```python
from build123d import *

# Parameters (mm, degrees)
SKETCH1_W           = 254
SKETCH1_H           = 177.8
BOSS_EXTRUDE1_DEPTH = 127
SKETCH2_W           = 228.6
SKETCH2_H           = 152.4
CUT_EXTRUDE1_DEPTH  = 101.6


with BuildPart() as part:
    # Sketch1 → Boss-Extrude1 (new body)
    with BuildSketch(Plane(origin=(0, 0, 0), x_dir=(1, 0, 0), z_dir=(0, 1, 0))):
        Rectangle(SKETCH1_W, SKETCH1_H)
    extrude(amount=BOSS_EXTRUDE1_DEPTH)

    # Sketch2 → Cut-Extrude1 (cut)
    with BuildSketch(Plane(origin=(0, 127, 0), x_dir=(1, 0, 0), z_dir=(0, 1, 0))):
        Rectangle(SKETCH2_W, SKETCH2_H)
    extrude(amount=-CUT_EXTRUDE1_DEPTH, mode=Mode.SUBTRACT)


solid = part.part
```
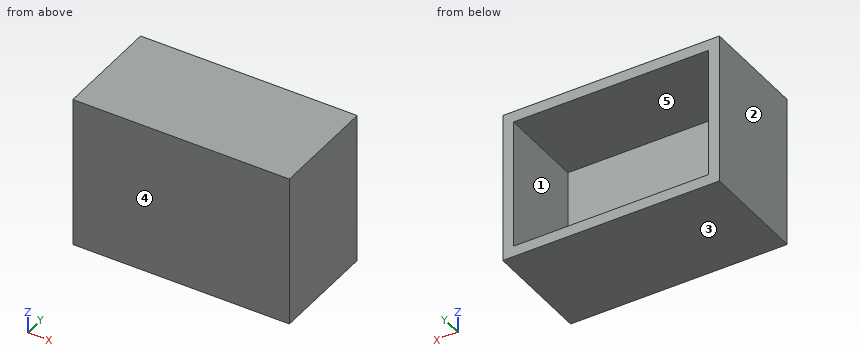
Read the model definition and answer for the solid it produces. Units are mm, in the model's axes. Face numbers are marked on the shaded views. A direction names the side the tool comes from. Round coordinates to 2 decimals unless told otherwise and drop trailing zeros. Write each loop counter-clockwise with the first axis right and the second up, starting at its lowest first coordinate (ties: lowest second). Pieces come first, ordered by that corner, then holes. Notation, with made-up numbers: M 42,-12.5 L 91,-12.5 A12 cw 91,-1.5 Z; hole C 21.5,-33.75 d10. An arc over 180 degrees is marked long. One line per item, written item: value.
Q1. Which of the six approach directions +Z, -Z, +X, -X, +Y, -Y give full straight-line access (tool end or side, diameter ignored) to the marked faces 4 and 5?
Data:
face 4: +Z, -Z, +X, -X, -Y
face 5: +Y
Q2. Find section A-A on y = 35. Write down the section's boundary in (x, z), plus the area to 3 significant figures.
Data:
outline: M -127,-88.9 L 127,-88.9 L 127,88.9 L -127,88.9 Z; hole M -114.3,-76.2 L 114.3,-76.2 L 114.3,76.2 L -114.3,76.2 Z
area: 10,300 mm2
Q3. For a pull along Z with two mould halves and no side action, classify the marked faces 1, 2 and 3 as +Z half, -Z half, draft (parallel to the pull), parting line (faces both ways), or undercut.
Data:
face 1: undercut
face 2: draft
face 3: -Z half
Q4. Find section C-C on z = -47.5. Write down the section's boundary in (x, y), plus the area to 3 significant figures.
Data:
outline: M -127,0 L 127,0 L 127,127 L 114.3,127 L 114.3,25.4 L -114.3,25.4 L -114.3,127 L -127,127 Z
area: 9,030 mm2
Q5. Straight lines are drawn through the part: line 1 (X direction, y = 92.5, z = -64.5); line 2 (Z direction, x = 0, y = 35.5); line 3 (Y direction, x = 101, z = -24). For each, find the intervals that lie inside material, in ascending order. Write a range as [from, to].
Data:
line 1: [-127, -114.3], [114.3, 127]
line 2: [-88.9, -76.2], [76.2, 88.9]
line 3: [0, 25.4]
Q6. Find section B-B on x = 3. Write down the section's boundary in (y, z).
Data:
outline: M 0,-88.9 L 127,-88.9 L 127,-76.2 L 25.4,-76.2 L 25.4,76.2 L 127,76.2 L 127,88.9 L 0,88.9 Z
Q7. A flat-ended cylindrical pin translates along its axis: pin 1 Ø3 at (x, z) = (-27, -53.5) entering from +Y. Find the tip coordinate at first contact, or state that the pin passes through.
Data:
pin 1: y = 25.4
